Answer from the drawing. Dimensions are ordinates in mm from the lowest x, y and z of the part. Coordinates: 2 decimals unless noted, no trailing zeros. Loops run counter-clockwise (first coordinate to the right, second up) from the corner with the lowest first, then second, coordinate; pieces in that order, holes last.
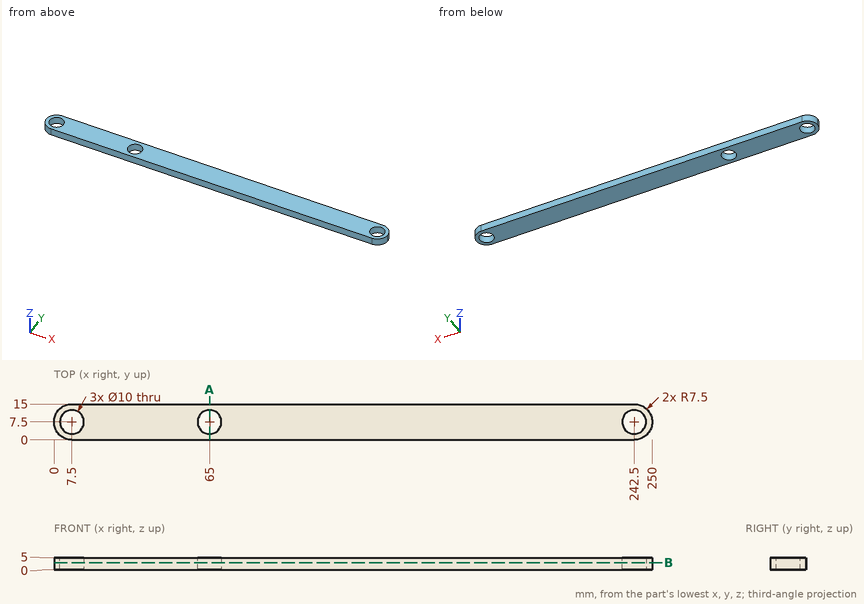
Item 1: Find the intervals of material crossed by line 1 along Y through (x, z) = (65, 2.15); line 2 along X through (y, z) = (6.25, 3.45); line 3 along X through (y, z) = (10, 4.2), in increasing order.
Numbers:
line 1: y = 0 to 2.5, 12.5 to 15
line 2: x = 0.1 to 2.66, 12.34 to 60.16, 69.84 to 237.66, 247.34 to 249.9
line 3: x = 0.43 to 3.17, 11.83 to 60.67, 69.33 to 238.17, 246.83 to 249.57
Item 2: A cutting plane is placed at A-A on x = 65. Determine the outline of the cut face in (y, z), then the cut area to 3 significant figures.
Numbers:
outline: (0, 0) - (2.5, 0) - (2.5, 5) - (0, 5) - close; (12.5, 0) - (15, 0) - (15, 5) - (12.5, 5) - close
area: 25.0 mm2
Item 3: A cutting plane is placed at B-B on z = 3. Determine the outline of the cut face in (x, y).
Numbers:
outline: (7.5, 0) - (242.5, 0) arc R7.5 ccw to (242.5, 15) - (7.5, 15) arc R7.5 ccw to start; hole circle Ø10 at (7.5, 7.5); hole circle Ø10 at (65, 7.5); hole circle Ø10 at (242.5, 7.5)
Item 4: Given pin 1 (2 mm diameter, centred on y = 2.5, z = 2, fed in from +X), flat-ended and moving along its own axis, determine where the tip first touches the part or whether it passes through.
Numbers:
pin 1: stops at x = 248.84
